CAD build for the part. Positions are in the model's coordinates, mm. Give positions to 0.01 mm unless a question says otherwise; leave off trailing zeros. Loops run counter-clockwise (first coordinate to the right, second up) from the corner with the lowest first, then second, coordinate; pieces in that order, holes last. Notation, with made-up numbers: M -10.5,-27.75 L 8.5,-27.75 A23 cw 8.5,-3.75 Z; hole C 24,-10 d1. An arc over 180 degrees is marked long. Answer as CSV lines item,"result".
```python
from build123d import *
from build123d import SkipClean  # not in build123d's __all__

# Parameters (mm, degrees)
F1_DEPTH = 6


with BuildPart() as f1:
    # F0 (on Front) → F1 (new body)
    with BuildSketch(Plane.XZ):
        with BuildLine():
            Line((-43, 0), (0, 0))
            Line((0, 0), (0, 81.5))
            ThreePointArc((0, 81.5), (-8.5, 90), (0, 98.5))
            Line((0, 98.5), (0, 115))
            ThreePointArc((0, 115), (-15.6853772226, 109.4671246306), (-24.4279354617, 95.3175153107))
            Line((-24.4279354617, 95.3175153107), (-43, 10))
            Line((-43, 10), (-43, 0))
        make_face()
    extrude(amount=F1_DEPTH)

    # F2: F1 across plane


with BuildPart() as f1_1:
    add(f1.part, clean=False)
    with SkipClean():  # cleaning this boolean's faces spoils the solid; the shape is the same uncleaned
        add(f1.part.mirror(Plane.YZ), clean=False)


solid = f1_1.part
```
Q1. Wall check: line 1 (Z direction, x = 0, y = -3.5); line 2 (X direction, y = -3.6, z = 90); line 3 (X direction, y = -3, z = 95). Give the ranges that are in metal, low to high. Write a range as [from, to].
Solution:
line 1,"z = [0, 81.5], [98.5, 115]"
line 2,"x = [-25.59, -8.5], [8.5, 25.59]"
line 3,"x = [-24.5, -6.87], [6.87, 24.5]"
Q2. Mould opens along X. For faces 1 (the flat face through (43, -3, 5)), 2 (the cylindrical face through (0.37, -2.96, 98.49)), 3 (the flat face through (1, -3, 0)) say: released by +X, released by -X, zero draft, split by the parting line, or undercut.
Solution:
face 1,"released by +X"
face 2,"undercut"
face 3,"zero draft"
Q3. Cut at A-A (y = -2). Write the cut outline in (x, z), and give its area (3 significant figures).
Solution:
outline,"M -43,0 L 43,0 L 43,10 L 24.43,95.32 A25 ccw -24.43,95.32 L -43,10 Z; hole C 0,90 d17"
area,"7,100 mm²"
Q4. Cut at D-D (x = 32). Write the cut outline in (y, z), and give its area (3 significant figures).
Solution:
outline,"M -6,0 L 0,0 L 0,60.53 L -6,60.53 Z"
area,"363 mm²"
Q5. Cut at C-C (z = 90). Write the cut outline in (x, y).
Solution:
outline,"M -25.59,-6 L -8.5,-6 L -8.5,0 L -25.59,0 Z; M 8.5,-6 L 25.59,-6 L 25.59,0 L 8.5,0 Z"
Q6. Pin check, flat tips, straight feed: P1, Ø1, axis at y = -1, z = 52, coming from the -X side; P2, Ø1.5, axis at x = -22.5, y = -5, coming from the +Z side; P3, Ø1.5, axis at x = -9, y = -2, coming from the +Z side. Stop position of each tip, or through.
Solution:
P1,"stops at x = -33.97"
P2,"stops at z = 102.33"
P3,"stops at z = 113.6"
Q7. Cut at B-B (x = -4). Write the cut outline in (y, z).
Solution:
outline,"M -6,0 L 0,0 L 0,82.5 L -6,82.5 Z; M -6,97.5 L 0,97.5 L 0,114.68 L -6,114.68 Z"
